Study the drawing (mm; zero at the part's minimum x, y, z) and answer. Coordinates: 2 decimals unless noted, no trailing zeros. Loops run counter-clockwise (first coordinate to the right, second up) from the corner with the lowest first, then second, coordinate; pieces in that order, holes last. Notation, with made-up numbers: (43, 0.5) -> (63, 0.5) arc R13 ccw to (63, 21.5) -> close; hole circle Ø9 at (70.25, 22). An arc over 180 degrees is marked (long way). Answer as a JSON object with one key per item and string values. Group by question number.
Q1. The part is cut by section A-A on y = 8.5. Write down the section's boundary in (x, z) (1 decimal).
Q2. This flat-tipped pin is pushed along its axis until it touches: P1, Ø1.8, axis at x = 25.13, z = 21.92, coming from the -Y side. Where does it stop, or does it pass through?
Q3. Determine the mould class of the marked faces 1, 2, 3 and 4 for opening direction Z: released by +Z, released by -Z, zero draft, split by the parting line, or undercut.
Q4. The part is cut by section D-D on y = 13. Write down the section's boundary in (x, z) (1 decimal).
Q5. The part is cut by section C-C on z = 5. Write down the section's boundary in (x, y).
Q6. Straight lines are drawn through the part: line 1 along Z through (x, y) = (25, 2) (1 decimal); line 2 along Z through (x, y) = (24.5, 8.5) (1 decimal); line 3 along X through (y, z) = (6.5, 6.5) (1 decimal). For each, find the intervals that lie inside material, in ascending order. Write a range as [from, to].
Q7. The part is cut by section B-B on x = 15. State how many separate pieces and enclosed holes the cut face has, and give its area (3 significant figures).
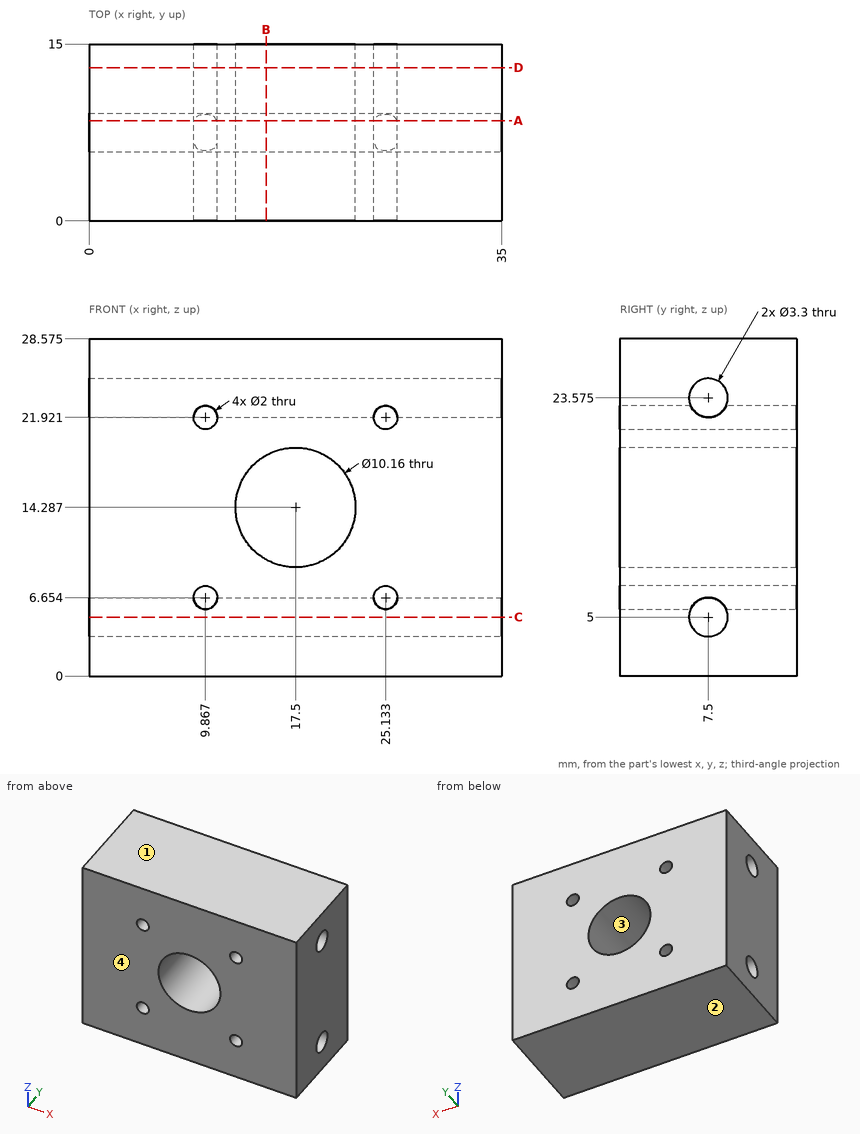
Final values:
{
 "1": {"outline": "(0, 0) -> (35, 0) -> (35, 3.7) -> (0, 3.7) -> close; (0, 6.3) -> (8.9, 6.3) arc R1 cw (long way) to (10.8, 6.3) -> (24.2, 6.3) arc R1 cw (long way) to (26.1, 6.3) -> (35, 6.3) -> (35, 22.3) -> (26.1, 22.3) arc R1 cw (long way) to (24.2, 22.3) -> (10.8, 22.3) arc R1 cw (long way) to (8.9, 22.3) -> (0, 22.3) -> close; (0, 24.9) -> (35, 24.9) -> (35, 28.6) -> (0, 28.6) -> close; hole circle Ø10.2 at (17.5, 14.3)"},
 "2": {"P1": "passes through"},
 "3": {"face 1": "released by +Z", "face 2": "released by -Z", "face 3": "undercut", "face 4": "zero draft"},
 "4": {"outline": "(0, 0) -> (35, 0) -> (35, 28.6) -> (0, 28.6) -> close; hole circle Ø2 at (9.9, 6.7); hole circle Ø2 at (9.9, 21.9); hole circle Ø10.2 at (17.5, 14.3); hole circle Ø2 at (25.1, 6.7); hole circle Ø2 at (25.1, 21.9)"},
 "5": {"outline": "(0, 0) -> (35, 0) -> (35, 5.85) -> (0, 5.85) -> close; (0, 9.15) -> (35, 9.15) -> (35, 15) -> (0, 15) -> close"},
 "6": {"line 1": "z = [0, 5.7], [7.6, 20.9], [22.9, 28.6]", "line 2": "z = [0, 3.7], [7.4, 21.1], [24.9, 28.6]", "line 3": "x = [0, 8.9], [10.9, 24.1], [26.1, 35]"},
 "7": {"separate pieces": "2", "enclosed holes": "2", "area": "279 mm2"}
}
